Geometry check sheet. Reference: the model listing, model coordinates, mm. A direction names the side the tool comes from. Coordinates: 2 decimals unless noted, no trailing zeros. Order: outer loops, then holes, each group sorted by start corner. A loop starts at its lowest first (then second) coordinate and runs counter-clockwise, first axis right, second up.
Autodesk Inventor part; units mm, degrees
ref_plane "YZ Plane" through (0, 0, 0) normal (1, 0, 0) x (0, 1, 0)
ref_plane "XZ Plane" through (0, 0, 0) normal (0, 1, 0) x (-1, 0, 0)
ref_plane "XY Plane" through (0, 0, 0) normal (0, 0, 1) x (1, 0, 0)
sketch "Sketch1" plane through (0, 0, 0) normal (0, 0, 1) x (1, 0, 0)
  line L0 (0, 0) -> (14.5304, 0)
  line L1 (-8.7854, 6.6412) -> (11.016, 6.6412)
  line L2 (11.016, 1.6412) -> (2.0946, 1.6412)
  line L3 (2.0946, 1.6412) -> (2.0946, -0.3588)
  line L4 (2.0946, -0.3588) -> (5.4596, -0.3588)
  line L5 (2.5721, -3.1588) -> (-3.1429, -3.1588)
  line L6 (-3.1429, -3.1588) -> (-6.0304, -1.1208)
  line L7 (-6.0304, -1.1208) -> (-6.0304, -0.3588)
  line L8 (-6.0304, -0.3588) -> (-2.6654, -0.3588)
  line L9 (-2.6654, -0.3588) -> (-2.6654, 1.6412)
  line L10 (-2.6654, 1.6412) -> (-8.7854, 1.6412)
  line L11 (-8.7854, 1.6412) -> (-8.7854, 6.6412)
  line L12 (5.4596, -0.3588) -> (5.4596, -1.1208)
  line L13 (5.4596, -1.1208) -> (2.5721, -3.1588)
  line L14 (11.016, 6.6412) -> (11.016, 1.6412)
  line L15 (0, 0) -> (0, 4.3587)
  line L16 (11.016, 6.6412) -> (11.016, 1.6412)
  dimension "d2" = 5
  dimension "d3" = 2
  dimension "d4" = 4.76
  dimension "d6" = 11.49
  dimension "d7" = 2.755
  dimension "d8" = 5.715
  dimension "d9" = 5.6425
  dimension "d10" = 6.12
  dimension "d11" = 0.762
  dimension "d12" = 0.762
  dimension "d50" = 144.786
  dimension "d51" = 2.8875
  dimension "d53" = 11.016
extrude "Extrusion1" add sketch "Sketch1" along normal blind 203.2
mirror "Mirror1" about plane through (11.016, 1.6412, 0) normal (1, 0, 0)
equation "\"d7\" = -0.5 * d6 + 0.5 * d0"
equation "\"d9\" = -0.5 * d8 + 0.5 * d0"
equation "\"d10\" = -0.5 * d4 + 0.5 * d0"
equation "\"d12\" = d11"
properties part number "Sliderfor2020"
Item 1: Thickness scan on line 1 along X through (y, z) = (0.5, 81); line 2 along Y through (x, z) = (-6, 182.5); line 3 along Y through (x, z) = (28.5, 74.5). Record the ranges inside material, lowest first.
Item 2: Release check for a two-part mould opening along X. For faces 4 (the face through (4, -0.359, 100)), 5 (the face through (11, 1.641, 100)), 6 (the face through (-8.785, 4, 100)), 7 (the face through (22, -3.159, 100)) record: pulls with the +X half, pulls with the -X half, needs draft (parallel to the pull), parting line crosses it, or undercut.
Item 3: Sectioned sample at B-B (x = 12). Record the cut outline in (y, z).
Item 4: Sectioned sample at A-A (z = 56.5). Record the cut outline in (x, y).
Item 5: Tool access check on faces 1 (the face through (18, -0.359, 100)), 2 (the face through (-4, -0.359, 100)), 3 (the face through (26, -0.359, 100)). Record the directions out of +Z, -Z, +X, -X, +Y, -Y that give a thin tool (end or side, any length) a straight path to the whole face; none if there is none.
Item 6: Depth check by flat-ended pin: P1, Ø3, axis at y = -0.5, z = 144, coming from the +X side; P2, Ø1.8, axis at x = -5, z = 61, coming from the -Y side; P3, Ø6.5, axis at x = 29, z = 131.5, coming from the -Y side. Enter the tip coordinate at first touch or a pass-through.
Geometry check:
1. line 1: x = -2.67 to 2.09, 19.94 to 24.7
1. line 2: y = -1.14 to -0.36, 1.64 to 6.64
1. line 3: y = 1.64 to 6.64
2. face 4: undercut
2. face 5: undercut
2. face 6: pulls with the -X half
2. face 7: needs draft
3. outline: (1.64, 0) - (6.64, 0) - (6.64, 203.2) - (1.64, 203.2) - close
4. outline: (-8.79, 1.64) - (-2.67, 1.64) - (-2.67, -0.36) - (-6.03, -0.36) - (-6.03, -1.12) - (-3.14, -3.16) - (2.57, -3.16) - (5.46, -1.12) - (5.46, -0.36) - (2.09, -0.36) - (2.09, 1.64) - (19.94, 1.64) - (19.94, -0.36) - (16.57, -0.36) - (16.57, -1.12) - (19.46, -3.16) - (25.17, -3.16) - (28.06, -1.12) - (28.06, -0.36) - (24.7, -0.36) - (24.7, 1.64) - (30.82, 1.64) - (30.82, 6.64) - (-8.79, 6.64) - close
5. face 1: +Z, -Z
5. face 2: +Z, -Z, -X
5. face 3: +Z, -Z, +X
6. P1: stops at x = 28.06
6. P2: stops at y = -2.48
6. P3: stops at y = -2.75
